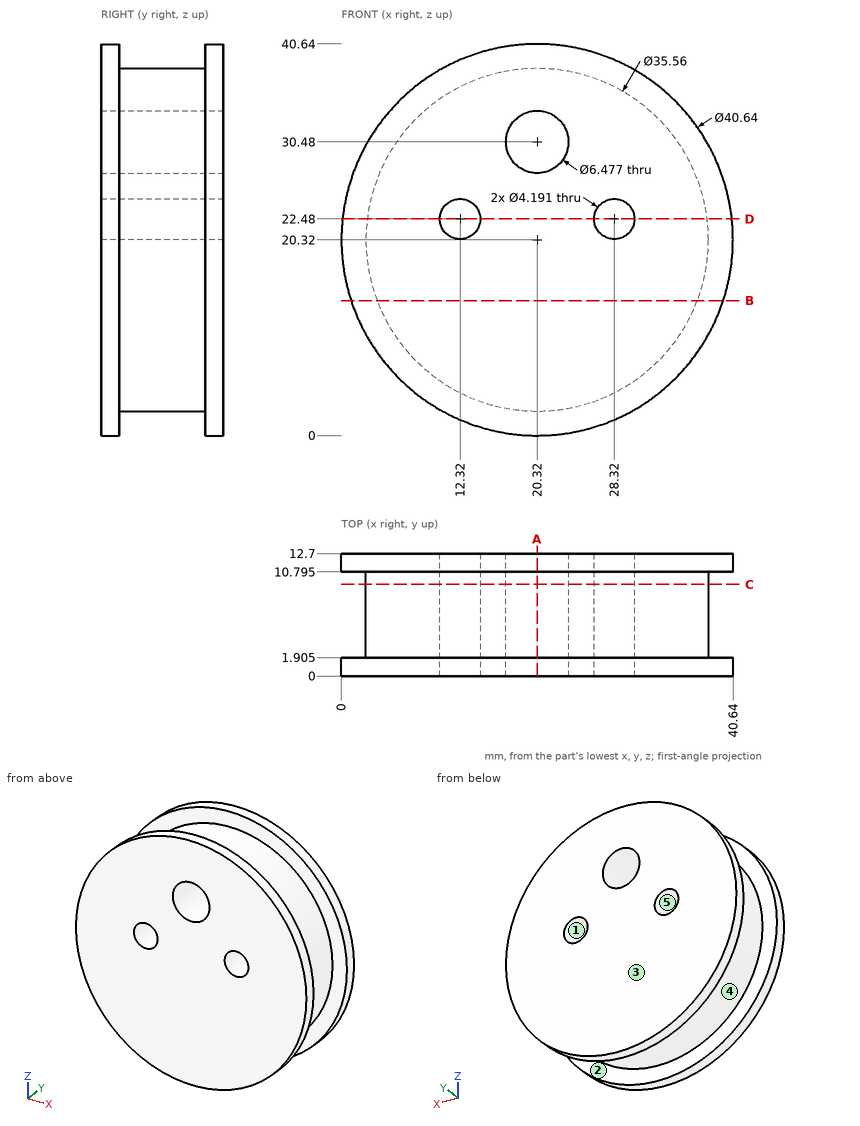
The drawing under review shows one solid part. Ordinate dimensions are in mm from its lowest x, y, z. A direction names the side the tool comes from. Give positions to 0.01 mm unless a question says otherwise; leave off trailing zeros. Order: outer loops, then holes, each group sorted by start corner. A loop starts at its lowest first (then second) coordinate and runs counter-clockwise, first axis right, second up. Notation, with made-up numbers: (88, -24) -> (93, -24) arc R16 ccw to (93, -2) -> close; hole circle Ø4 at (38.5, 66). An arc over 180 degrees is marked (long way). Write item = value, one per line.
1) For the marked faces 1 and 2, list the 3-axis set-ups (+Z, -Z, +X, -X, +Y, -Y) from which the entire face can be reached by the end or side of a thin tool; tool diameter is ignored.
Findings:
face_1 = +Y, -Y
face_2 = none
2) We need section A-A, the plane x = 20.32. Give the boundary of the cut face in (y, z) (1 decimal).
Findings:
outline = (0, 0) -> (1.9, 0) -> (1.9, 2.5) -> (10.8, 2.5) -> (10.8, 0) -> (12.7, 0) -> (12.7, 27.2) -> (0, 27.2) -> close; (0, 33.7) -> (12.7, 33.7) -> (12.7, 40.6) -> (10.8, 40.6) -> (10.8, 38.1) -> (1.9, 38.1) -> (1.9, 40.6) -> (0, 40.6) -> close
3) We need section D-D, the plane z = 22.48. Give the boundary of the cut face in (x, y) (1 decimal).
Findings:
outline = (0.1, 0) -> (10.2, 0) -> (10.2, 12.7) -> (0.1, 12.7) -> (0.1, 10.8) -> (2.7, 10.8) -> (2.7, 1.9) -> (0.1, 1.9) -> close; (14.4, 0) -> (26.2, 0) -> (26.2, 12.7) -> (14.4, 12.7) -> close; (30.4, 0) -> (40.5, 0) -> (40.5, 1.9) -> (38, 1.9) -> (38, 10.8) -> (40.5, 10.8) -> (40.5, 12.7) -> (30.4, 12.7) -> close
4) We need section C-C, the plane y = 9.5. Give the boundary of the cut face in (x, z), and give its area (3 significant figures).
Findings:
outline = circle Ø35.56 at (20.32, 20.32); hole circle Ø4.19 at (12.32, 22.48); hole circle Ø6.48 at (20.32, 30.48); hole circle Ø4.19 at (28.32, 22.48)
area = 933 mm^2
5) Insertion check: pin 1 (5 mm diameter, centred on x = 4.5, y = 9, fed in from +Z); pin 2 (6 mm diameter, centred on y = 3, z = 4, fed in from -X); pin 3 (5 mm diameter, centred on y = 7.5, z = 26.5, fed in from +X) (3 decimals); pin 4 (20.5 mm diameter, centred on x = 27, z = 22, fed in from +Y). Each pin has a flat end and moves straight along its axis. Give the tip position at first contact, or say it passes through.
Findings:
pin_1 = 34.97
pin_2 = 5.16
pin_3 = 37.715
pin_4 = 12.7
6) To check wall thickness, follow L1, parallel to X at y = 8.25, z = 22.48; L2, parallel to X at y = 6.5, z = 21; L3, parallel to Z at x = 20.32, y = 6.75. State the ranges of each line that lie inside material, in increasing order. Write a range as from..to.
Findings:
L1 = 2.67..10.22, 14.42..26.22, 30.42..37.97
L2 = 2.55..10.84, 13.8..26.84, 29.8..38.09
L3 = 2.54..27.24, 33.72..38.1
7) Draft analysis for pull direction X (two halves, no side actions). For the marked faces 3, 4 and 5, state which applies: pulls with the +X half, pulls with the -X half, needs draft (parallel to the pull), parting line crosses it, or undercut.
Findings:
face_3 = needs draft
face_4 = parting line crosses it
face_5 = undercut
8) We need section B-B, the plane z = 14. Give the boundary of the cut face in (x, y) (3 decimals), and give its area (3 significant figures).
Findings:
outline = (1.008, 0) -> (39.632, 0) -> (39.632, 1.905) -> (36.939, 1.905) -> (36.939, 10.795) -> (39.632, 10.795) -> (39.632, 12.7) -> (1.008, 12.7) -> (1.008, 10.795) -> (3.701, 10.795) -> (3.701, 1.905) -> (1.008, 1.905) -> close
area = 443 mm^2
